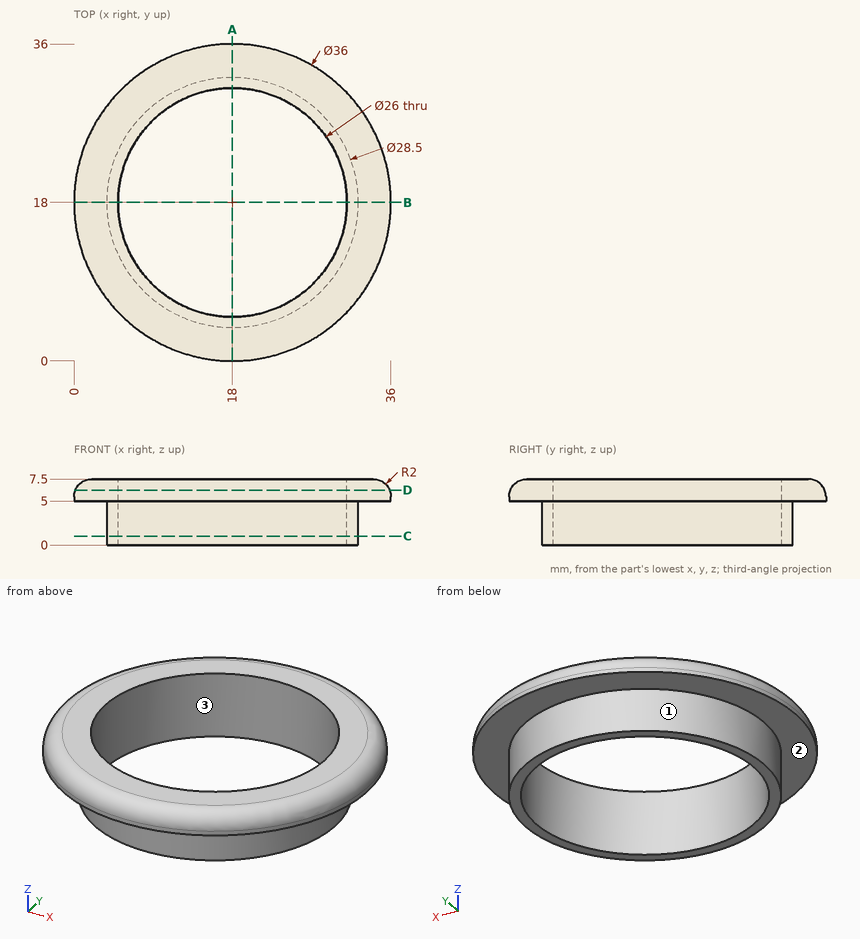
Here's the drawing with two shaded views (mm, measured from the low corner). I have some questions. Coordinates: 2 decimals unless noted, no trailing zeros. Loops run counter-clockwise (first coordinate to the right, second up) from the corner with the lowest first, then second, coordinate; pieces in that order, holes last. Notation, with made-up numbers: (59, -39) -> (94, -39) arc R18 cw to (94, -6) -> close; hole circle Ø10 at (38, 8). An arc over 180 degrees is marked (long way). Put each result on its own line as item: value. Start each with the question number.
Q1. If I drill on line 1 (Y direction, x = 18, z = 4.75); line 2 (Z direction, x = 26, y = 5), over which ranges is the centre line in solid material (lowest first)? Write a range as [from, to].
Q2. I want a section at C-C (z = 1). Write out the boundary of the cut face in (x, y), plus the area to 3 significant figures.
Q3. I'm going to push flat-ended pins straight in: P1, Ø1.5, axis at x = 20, z = 6.5, coming from the +Y side; P2, Ø1.5, axis at y = 18.5, z = 1.5, coming from the -X side; P3, Ø1.5, axis at y = 23.5, z = 5.5, coming from the -X side. Where does each tip first touch, or does it pass through?
Q4. I want a section at A-A (x = 18). Write out the boundary of the cut face in (y, z).
Q5. Thinking about a two-plate mould opening in X: for the marked faces 1, 2 and 3, which applies, pulls with the +X half, pulls with the -X half, needs draft (parallel to the pull), parting line crosses it, or undercut?
Q6. I want a section at D-D (z = 6.25). Write out the boundary of the cut face in (x, y).
Taken from the geometry:
1. line 1: y = [3.75, 5], [31, 32.25]
1. line 2: z = [5, 7.5]
2. outline: circle Ø28.5 at (18, 18); hole circle Ø26 at (18, 18)
2. area: 107 mm2
3. P1: stops at y = 35.9
3. P2: stops at x = 3.75
3. P3: stops at x = 0.64
4. outline: (0, 5) -> (3.75, 5) -> (3.75, 0) -> (5, 0) -> (5, 7.5) -> (2, 7.5) arc R2 ccw to (0, 5.5) -> close; (31, 0) -> (32.25, 0) -> (32.25, 5) -> (36, 5) -> (36, 5.5) arc R2 ccw to (34, 7.5) -> (31, 7.5) -> close
5. face 1: parting line crosses it
5. face 2: needs draft
5. face 3: undercut
6. outline: circle Ø35.71 at (18, 18); hole circle Ø26 at (18, 18)
